Answer from the drawing. Dimensions are ordinates in mm from the lowest x, y and z of the part. Coordinates: 2 decimals unless noted, no trailing zeros. Write each loop counter-clockwise with the first axis right and the second up, starting at its lowest first coordinate (ties: lowest second). Pieces come first, ordered by that corner, then holes.
(1) Straight lines are drawn through the part: line 1 (Y direction, x = 35.6, z = 32); line 2 (Y direction, x = 6, z = 23.5); line 3 (X direction, y = 65, z = 21). For each, find the intervals that lie inside material, in ascending order.
(2) The part is cut by section A-A on y = 35.6. Determine the outline of the cut face in (x, z).
(3) Given P1, Ø8, axis at x = 65.2, y = 35.6, coming from the +Z side; P2, Ø4, axis at x = 8.5, z = 10, coming from the +Y side; P3, Ø6, axis at y = 58, z = 21, coming from the +X side; P4, Ø3, axis at y = 15, z = 23.5, coming from the -X side, each flat-ended and moving along its own axis, determine where each tip first touches the part or whether it passes through.
(4) The part is cut by section C-C on y = 6. Determine the outline of the cut face in (x, z).
(5) For a pull along X with two mould halves and no side action, classify the marked faces 1, 2, 3 and 4 as +X half, -X half, draft (parallel to the pull), parting line (faces both ways), or undercut.
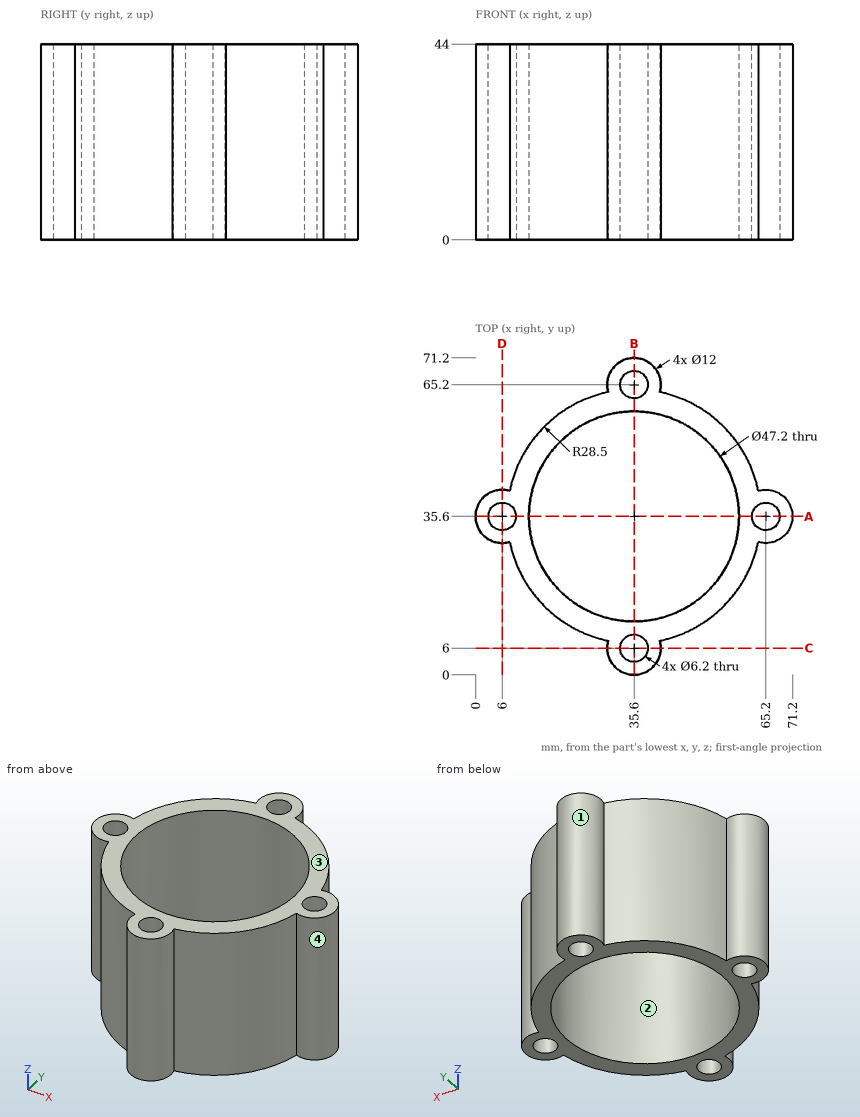
Model answer:
1. line 1: y = 0 to 2.9, 9.1 to 12, 59.2 to 62.1, 68.3 to 71.2
1. line 2: y = 29.6 to 32.5, 38.7 to 41.6
1. line 3: x = 29.6 to 32.51, 38.69 to 41.6
2. outline: (0, 0) - (2.9, 0) - (2.9, 44) - (0, 44) - close; (9.1, 0) - (12, 0) - (12, 44) - (9.1, 44) - close; (59.2, 0) - (62.1, 0) - (62.1, 44) - (59.2, 44) - close; (68.3, 0) - (71.2, 0) - (71.2, 44) - (68.3, 44) - close
3. P1: stops at z = 44
3. P2: stops at y = 49.1
3. P3: stops at x = 56.48
3. P4: stops at x = 14.45
4. outline: (29.6, 0) - (32.5, 0) - (32.5, 44) - (29.6, 44) - close; (38.7, 0) - (41.6, 0) - (41.6, 44) - (38.7, 44) - close
5. face 1: parting line
5. face 2: undercut
5. face 3: draft
5. face 4: undercut
